The drawing under review shows one solid part. Ordinate dimensions are in mm from its lowest x, y, z. A direction names the side the tool comes from. Coordinates: 2 decimals unless noted, no trailing zeros. Order: outer loops, then holes, each group sorted by start corner. A loop starts at its lowest first (then second) coordinate and runs counter-clockwise, first axis right, second up. Notation, with made-up numbers: (87, 31.5) -> (104, 31.5) arc R8 ccw to (104, 46.5) -> close; hole circle Ø6 at (-1.75, 69.5). An arc over 180 degrees is marked (long way). Use one line per item in the form item = value.
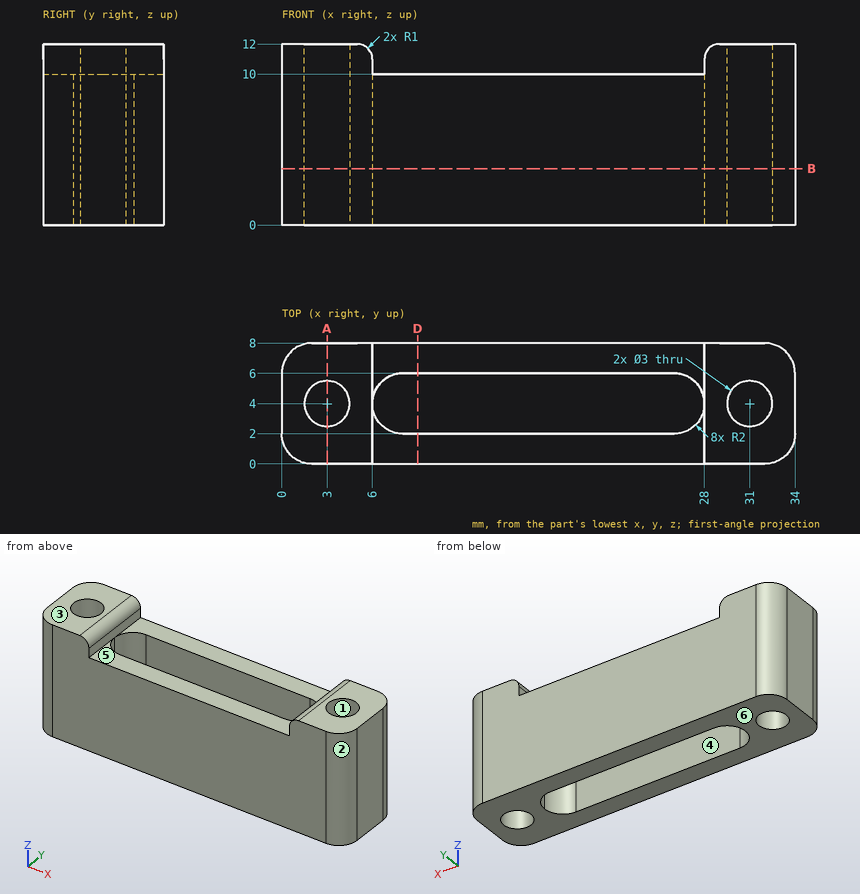
Item 1: To check wall thickness, follow L1, parallel to Y at x = 23, z = 8.25; L2, parallel to X at y = 4.5, z = 4.5 (1 decimal); L3, parallel to Z at x = 22, y = 7.75. State the ranges of each line that lie inside material, in increasing order. Write a range as from..to.
Results found:
L1 = 0..2, 6..8
L2 = 0..1.6, 4.4..6.1, 27.9..29.6, 32.4..34
L3 = 0..10
Item 2: We need section A-A (x = 3). Write out the cut boundary in (y, z), plus the area to 3 significant figures.
Results found:
outline = (0, 0) -> (2.5, 0) -> (2.5, 12) -> (0, 12) -> close; (5.5, 0) -> (8, 0) -> (8, 12) -> (5.5, 12) -> close
area = 60.0 mm²
Item 3: We need section B-B (z = 3.75). State how many separate pieces and enclosed holes the cut face has, plus the area to 3 significant figures.
Results found:
separate_pieces = 1
enclosed_holes = 3
area = 170 mm²
Item 4: Draft analysis for pull direction Y (two halves, no side actions). For the marked faces 1, 2 and 3, state which applies: released by +Y, released by -Y, zero draft, split by the parting line, or undercut.
Results found:
face_1 = undercut
face_2 = released by -Y
face_3 = zero draft
Item 5: We need section D-D (x = 9). Write out the cut boundary in (y, z), plus the area to 3 significant figures.
Results found:
outline = (0, 0) -> (2, 0) -> (2, 10) -> (0, 10) -> close; (6, 0) -> (8, 0) -> (8, 10) -> (6, 10) -> close
area = 40.0 mm²
Item 6: Clearance check with flat-ended pins moving along their axes: pin 1 (3 mm diameter, centred on x = 14.5, z = 5, fed in from -Y); pin 2 (2.5 mm diameter, centred on x = 31, y = 4, fed in from +Z); pin 3 (2 mm diameter, centred on x = 12, y = 6, fed in from +Z). State where each tip first meets the part, or that it passes through.
Results found:
pin_1 = 0
pin_2 = through
pin_3 = 10
Item 7: Tool access review of the marked faces 4, 5 and 6: name each direction out of +Z, -Z, +X, -X, +Y, -Y from which nothing blocks a thin tool from reaching the whole face with its end or side.
Results found:
face_4 = +Z, -Z
face_5 = +Z, +Y, -Y
face_6 = -Z, +X, -X, +Y, -Y
